Verification items for the finished model (mm, model axes). Face numbers are marked on the shaded views. A direction names the side the tool comes from. Coordinates: 2 decimals unless noted, no trailing zeros. Order: outer loops, then holes, each group sorted by start corner. A loop starts at its lowest first (then second) coordinate and runs counter-clockwise, first axis right, second up. Notation, with made-up numbers: M -37,66 L 20,66 A17 cw 20,71 Z; hole C 64.5,46 d3. An arc over 180 degrees is marked long. Answer as a JSON object with one key per item and string values. Group by question number.
(1) Access from +Z, -Z, +X, -X, +Y, -Y to the whole of each face (thin tool, end or side, straight path). Record for the marked faces 4, 5 and 6.
(2) Cross-section at C-C (z = -7.25). Enter the section's corners in (x, y).
(3) Material ranges on line 1 (X direction, y = -6.95, z = -4.35); line 2 (X direction, y = -11.3, z = -4.35); line 3 (Z direction, x = -48.75, y = -8), recorded low to high.
(4) Cross-section at B-B (x = -45.5). Enter the section's corners in (y, z).
(5) Cross-section at A-A (y = -10). Enter the section's corners in (x, z).
(6) Gauge pin test, flat ends, axial feed: pin 1 Ø0.9 at (y, z) = (-6.5, -7.5) entering from +X; pin 2 Ø1.4 at (y, z) = (-7, -8.5) entering from -X; pin 3 Ø3 at (y, z) = (-8, -9.5) entering from +X; pin 4 Ø2 at (x, z) = (-50, -4.35) entering from +Y. Record the tip position at first contact, or that the pin passes through.
(7) Mould release check, pull along X, two halves, no side actions. Record for the marked faces 1, 2 and 3: released by +X, released by -X, zero draft, split by the parting line, or undercut.
(8) Cross-section at D-D (x = -50.75). Enter the section's corners in (y, z).
Autodesk Inventor part; units mm, degrees
ref_plane "Arbeitsebene2" through (-53, -5.4, -13.5) normal (0, 0, -1) x (0, 1, 0)
ref_plane "YZ Plane" through (0, 0, 0) normal (1, 0, 0) x (0, 1, 0)
ref_plane "XZ Plane" through (0, 0, 0) normal (0, 1, 0) x (-1, 0, 0)
ref_plane "Arbeitsebene1" through (0, 0, 0) normal (0, 0, 1) x (1, 0, 0)
sketch "Skizze1" plane through (0, 0, 0) normal (0, 0, 1) x (1, 0, 0)
  arc A0 (-53, 5.4) -> (-47.2, -0.4) centre (-47.2, 5.4) ccw
  line L0 (-53, -5.4) -> (-53, 5.4)
  line L1 (-35.6871, -5.4) -> (-53, -5.4)
  line L2 (-35.6871, -0.4) -> (-35.6871, -5.4)
  line L3 (-47.2, -0.4) -> (-35.6871, -0.4)
  line L4 (-67.0006, -5.9) -> (-67.0006, -9.9)
  line L5 (-31.7506, -5.4) -> (-31.7506, -10.4)
  line L6 (-33.0006, -5.9) -> (-33.0006, -9.9) construction
  line L7 (-32.5561, -5.4) -> (-32.5561, -10.4)
  line L8 (-51.4006, -5.4) -> (-51.4006, 4.6)
  line L9 (-48.6006, -5.4) -> (-48.6006, 2.412)
  line L10 (-35.6871, -5.4) -> (-53.0408, -5.4)
  line L11 (-53.0408, -5.4) -> (-53.0408, -8.4)
  line L12 (-53.0408, -8.4) -> (-37.6871, -8.4)
  line L13 (-37.6871, -8.4) -> (-37.6871, -5.4)
  line L14 (-53.0408, -8.4) -> (-55.0408, -11.8641)
  line L15 (-53.0408, -8.4) -> (-49.0408, -8.4) construction
  line L16 (-55.0408, -11.8641) -> (-35.6871, -11.8641)
  line L17 (-35.6871, -11.8641) -> (-37.6871, -8.4)
  point P0 (0, 0)
  dimension "d0" = 3
  dimension "d1" = 4
  dimension "d2" = 120
  dimension "d3" = 60
  dimension "d14" = 2
ref_plane "Arbeitsebene2" through (-53, -5.4, -13.5) normal (0, 0, -1) x (0, 1, 0)
extrude "Extrusion1" add sketch "Skizze1" against normal up to surface (13.5 mm away) contours L1 L13 L12 L11 L10 | L12 L17 L16 L14
fillet "Rundung1" radius 0.5 4 edges at (-55.0408, -11.8641, -6.75) (-35.6871, -11.8641, -6.75) (-53.0408, -8.4, -6.75) (-37.6871, -8.4, -6.75)
sketch "Skizze2" plane through (-54.1748, -11.8641, 0) normal (0, -1, 0) x (1, 0, 0)
  circle A0 centre (9.8312, -6.75) radius 1.4
  circle A1 centre (4.1742, -4.35) radius 1.4
  line L0 (-0.6431, -6.75) -> (20.1351, -6.75)
  circle A2 centre (4.1742, -9.15) radius 1.4
  point P0 (54.1748, 0)
hole "Bohrung1" at (-50.0006, -11.8641, -4.35) at (-44.3436, -11.8641, -6.75) at (-50.0006, -11.8641, -9.15) direction (0, 1, 0) diameter 2.8 depth 14 tip angle 118 counterbore diameter 6.5 counterbore depth 3
properties part number "10_Cassete_Slide"
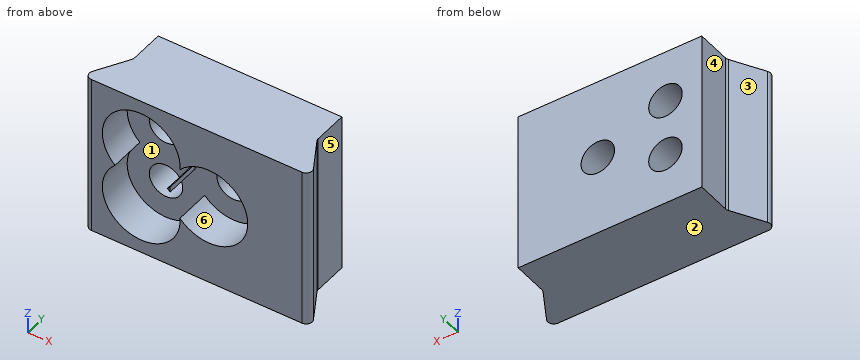
Taken from the geometry:
{
 "1": {"face 4": "+Z, -Z, -X, +Y", "face 5": "+Z, -Z, +X, +Y", "face 6": "-Y"},
 "2": {"outline": "M -54.61,-11.11 A0.5 ccw -54.17,-11.86 L -52.64,-11.86 L -52.64,-8.86 L -45.65,-8.86 L -45.65,-5.4 L -53.04,-5.4 L -53.04,-8.27 A0.5 cw -53.11,-8.52 Z; M -43.04,-8.86 L -41.13,-8.86 L -41.13,-11.86 L -36.55,-11.86 A0.5 ccw -36.12,-11.11 L -37.62,-8.52 A0.5 cw -37.69,-8.27 L -37.69,-5.4 L -43.04,-5.4 Z"},
 "3": {"line 1": "x = -53.04 to -51.4, -48.6 to -37.69", "line 2": "x = -54.67 to -53.25, -46.75 to -46.54, -42.15 to -36.06", "line 3": "z = -13.5 to -9.78, -8.52 to -4.98, -3.72 to 0"},
 "4": {"outline": "M -11.86,-13.5 L -5.4,-13.5 L -5.4,-7.54 L -8.86,-7.54 L -8.86,-9.79 L -11.86,-9.79 Z; M -11.86,-3.71 L -8.86,-3.71 L -8.86,-5.96 L -5.4,-5.96 L -5.4,0 L -11.86,0 Z"},
 "5": {"outline": "M -53.96,-13.5 L -36.76,-13.5 L -36.76,0 L -53.96,0 Z; M -47.81,-6.75 A3.25 cw -47.59,-6.97 A3.25 cw -47.59,-6.53 A3.25 cw Z; hole M -52.19,-6.75 A3.25 ccw long -46.76,-8.93 A3.25 ccw long -46.76,-4.57 A3.25 ccw long Z"},
 "6": {"pin 1": "stops at x = -37.69", "pin 2": "stops at x = -53.04", "pin 3": "stops at x = -37.05", "pin 4": "passes through"},
 "7": {"face 1": "undercut", "face 2": "zero draft", "face 3": "released by -X"},
 "8": {"outline": "M -11.86,-13.5 L -5.4,-13.5 L -5.4,-10.33 L -8.86,-10.33 L -8.86,-12.31 L -11.86,-12.31 Z; M -11.86,-1.19 L -8.86,-1.19 L -8.86,-3.17 L -5.4,-3.17 L -5.4,0 L -11.86,0 Z; M -8.86,-7.97 L -5.4,-7.97 L -5.4,-5.53 L -8.86,-5.53 Z"}
}
